Input: part model. Units: mm. Frame: model coordinates. A direction names the side the tool comes from. Round coordinates to 2 decimals unless told otherwise and drop trailing zeros. Loops run counter-clockwise (first coordinate to the right, second up) from the corner with the lowest first, then second, coordinate; pieces in that order, holes last. Notation, with made-up numbers: (17.25, 3) -> (63.25, 3) arc R16 ccw to (63.25, 28) -> close; hole circle Ø2 at (75.25, -24.75). An arc over 180 degrees is marked (long way). Answer as a JSON object with one key per item and string values. Group by question number.
Item 1: Material intervals for line 1 (Z direction, x = -14, y = 27); line 2 (Y direction, x = 29, z = 37); line 3 (Y direction, x = -27, z = 37), sorted ascending. Write a range as [from, to].
Item 2: Section query A-A on z = 13.5. Return loops of the section in (x, y) (1 decimal).
Item 3: Draft query along Y for faces 3 (the cylindrical face through (25.164, 0.441, 46.033)), 4 (the flat face through (2, -6, 44.45)), 5 (the flat face through (2, -6, 0)), 6 (the cylindrical face through (29.7, 1.9, 46)). Return one class per face: released by +Y, released by -Y, zero draft, split by the parting line, or undercut.
Item 4: Set-up query: faces 1 (the flat face through (25, -19, 47.625)), 2 (the flat face through (20, -33, 44.45)). Return all of +Z, -Z, +X, -X, +Y, -Y with unobstructed straight access to the full face (end or side cutting, diameter ignored); none if empty.
Item 5: Pin query (flat end, axial travel): pin 1 (1 mm diameter, centred on x = -13, z = 42.5, fed in from -Y); pin 2 (10 mm diameter, centred on y = -24.5, z = 18.5, fed in from -X); pin 3 (22.5 mm diameter, centred on x = 10.5, y = -10, fed in from +Z). Return the tip coordinate at first contact, or that it passes through.
from build123d import *

# Parameters (mm, degrees)
F1_DEPTH = 44.45
F2_R     = 28.575
F2_R_2   = 23.8125
F3_DEPTH = 3.175
F4_R     = 1.27


with BuildPart() as f1:
    # F0 (on Top) → F1 (new body)
    with BuildSketch(Plane.XY):
        with BuildLine():
            Line((42.139101, -46.398989), (42.139101, -6.711489))
            ThreePointArc((42.139101, -6.711489), (30.514902, -34.774789), (2.451601, -46.398989))
            Line((2.451601, -46.398989), (42.139101, -46.398989))
        make_face()
        with BuildLine():
            ThreePointArc((2.451601, -46.398989), (30.514902, -34.774789), (42.139101, -6.711489))
            ThreePointArc((42.139101, -6.711489), (-25.611699, 21.351812), (2.451601, -46.398989))
        make_face()
    extrude(amount=F1_DEPTH)

    # F2 (on face) → F3 (join)
    with BuildSketch(Plane.XY.offset(44.45)):
        with Locations((2.451601, -6.711489)):
            Circle(F2_R)
        with Locations((2.451601, -6.711489)):
            Circle(F2_R_2, mode=Mode.SUBTRACT)
    extrude(amount=F3_DEPTH)

    # F4
    f4_edges = [f1.edges().sort_by_distance(p)[0] for p in [
        (-26.123399, -6.711489, 47.625),
        (-21.360899, -6.711489, 47.625),
        (-26.123399, -6.711489, 44.45),
        (-21.360899, -6.711489, 44.45),
    ]]
    fillet(f4_edges, radius=F4_R)


solid = f1.part
Solved:
{
 "1": {"line 1": "[0, 44.45]", "line 2": "[-46.4, 22.79]", "line 3": "[-33.31, 19.89]"},
 "2": {"outline": "(2.5, -46.4) -> (42.1, -46.4) -> (42.1, -6.7) arc R39.7 ccw (long way) to start"},
 "3": {"face 3": "undercut", "face 4": "undercut", "face 5": "zero draft", "face 6": "split by the parting line"},
 "4": {"face 1": "+Z, +X, -X, +Y, -Y", "face 2": "+Z"},
 "5": {"pin 1": "y = -43.47", "pin 2": "x = -35.12", "pin 3": "z = 44.45"}
}
